For this review, take the finished solid that the model builds, in its own axes (mm). Give positions to 0.01 mm unless a question says otherwise; leave off trailing zeros. Order: outer loops, then holes, each group sorted by start corner. A loop starts at its lowest first (then second) coordinate and runs counter-clockwise, first axis right, second up. Notation, with made-up numbers: (37, 66) -> (44, 66) arc R18 cw to (44, 77) -> close; hole circle Ø3 at (67.5, 24). An arc over 180 degrees is marked (long way). Return JSON: item names as keys, results as strings. Group by question number.
1) Add section A-A (x = 4). Give the boundary of the cut face in (y, z).
2) Add section D-D (z = 2.75). Give the boundary of the cut face in (x, y).
3) Insertion check: P1, Ø3, axis at x = 3, y = 37.5, coming from the -Z side; P2, Ø3.5, axis at x = 38.5, y = 4, coming from the +Z side. Each pin has a flat end and moves straight along its axis. Give the tip position at first contact, or say it passes through.
4) Add section B-B (y = 38.5). Give the boundary of the cut face in (x, z), then the cut area to 3 significant figures.
5) Add section C-C (x = 47). Give the boundary of the cut face in (y, z), then the cut area to 3 significant figures.
6) To check wall thickness, follow line 1 along X through (y, z) = (4, 6.7); line 2 along X through (y, z) = (4, 5.55); line 3 along X through (y, z) = (38.5, 6.1). State the ranges of each line that lie inside material, in increasing order.
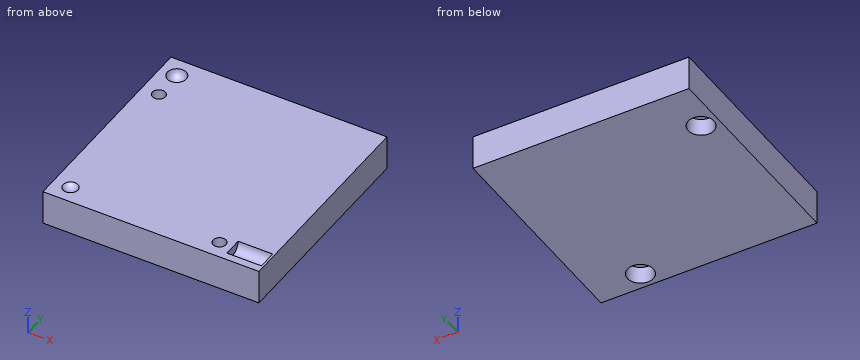
from build123d import *

# Parameters (mm, degrees)
CYLINDER012_R     = 2.2
CYLINDER012_DEPTH = 8
CYLINDER011_R     = 3
CYLINDER011_DEPTH = 4
CYLINDER010_R     = 1.5
CYLINDER010_DEPTH = 8
CYLINDER009_R     = 3
CYLINDER009_DEPTH = 4
CYLINDER008_R     = 1.5
CYLINDER008_DEPTH = 8
BOX002_W          = 50
BOX002_H          = 50
BOX002_DEPTH      = 8


with BuildPart() as cylinder012:
    # Cylinder012 → Cylinder012 (new body)
    with BuildSketch(Plane(origin=(41.5, 4, 8), x_dir=(0, 0, -1), z_dir=(1, 0, 0))):
        Circle(CYLINDER012_R)
    extrude(amount=CYLINDER012_DEPTH)


with BuildPart() as sphere003:
    # Sphere003 → Sphere003 (revolve)
    with BuildSketch(Plane(origin=(4, 45.5, 8.1), x_dir=(1, 0, 0), z_dir=(0, -1, 0))):
        with BuildLine():
            ThreePointArc((0, -2.2), (2.2, 0), (0, 2.2))
            Line((0, 2.2), (0, -2.2))
        make_face()
    revolve(axis=Axis((4, 45.5, 8.1), (0, 0, 1)))


with BuildPart() as sphere001:
    # Sphere001 → Sphere001 (revolve)
    with BuildSketch(Plane(origin=(4, 4, 9), x_dir=(1, 0, 0), z_dir=(0, -1, 0))):
        with BuildLine():
            ThreePointArc((0, -2), (2, 0), (0, 2))
            Line((0, 2), (0, -2))
        make_face()
    revolve(axis=Axis((4, 4, 9), (0, 0, 1)))


with BuildPart() as cylinder011:
    # Cylinder011 → Cylinder011 (new body)
    with BuildSketch(Plane.XY):
        Circle(CYLINDER011_R)
    extrude(amount=CYLINDER011_DEPTH)


with BuildPart() as springhole004:
    # Cylinder010 → Cylinder010 (new body)
    with BuildSketch(Plane.XY):
        Circle(CYLINDER010_R)
    extrude(amount=CYLINDER010_DEPTH)

    # Fusion005: union Cylinder011
    add(cylinder011.part)


with BuildPart() as springhole004_1:
    # Fusion005 placement: moved
    add(springhole004.part.moved(Location((4, 38.5, 0))))


with BuildPart() as cylinder009:
    # Cylinder009 → Cylinder009 (new body)
    with BuildSketch(Plane.XY):
        Circle(CYLINDER009_R)
    extrude(amount=CYLINDER009_DEPTH)


with BuildPart() as springhole003:
    # Cylinder008 → Cylinder008 (new body)
    with BuildSketch(Plane.XY):
        Circle(CYLINDER008_R)
    extrude(amount=CYLINDER008_DEPTH)

    # Fusion004: union Cylinder009
    add(cylinder009.part)


with BuildPart() as springhole003_1:
    # Fusion004 placement: moved
    add(springhole003.part.moved(Location((38.5, 4, 0))))


with BuildPart() as cut012:
    # Box002 → Box002 (new body)
    with BuildSketch(Plane.XY):
        with Locations((25, 25)):
            Rectangle(BOX002_W, BOX002_H)
    extrude(amount=BOX002_DEPTH)

    # Cut008: cut SpringHole003
    add(springhole003_1.part, mode=Mode.SUBTRACT)

    # Cut009: cut SpringHole004
    add(springhole004_1.part, mode=Mode.SUBTRACT)

    # Cut010: cut Sphere001
    add(sphere001.part, mode=Mode.SUBTRACT)

    # Cut011: cut Sphere003
    add(sphere003.part, mode=Mode.SUBTRACT)

    # Cut012: cut Cylinder012
    add(cylinder012.part, mode=Mode.SUBTRACT)


solid = cut012.part
Evaluation:
{
 "1": {"outline": "(0, 0) -> (35.5, 0) -> (35.5, 4) -> (37, 4) -> (37, 8) -> (5.73, 8) arc R2 cw to (2.27, 8) -> (0, 8) -> close; (40, 4) -> (41.5, 4) -> (41.5, 0) -> (50, 0) -> (50, 8) -> (47.7, 8) arc R2.2 cw to (43.3, 8) -> (40, 8) -> close"},
 "2": {"outline": "(0, 0) -> (50, 0) -> (50, 50) -> (0, 50) -> close; hole circle Ø6 at (4, 38.5); hole circle Ø6 at (38.5, 4)"},
 "3": {"P1": "z = 4", "P2": "z = 8"},
 "4": {"outline": "(0, 0) -> (1, 0) -> (1, 4) -> (2.5, 4) -> (2.5, 8) -> (0, 8) -> close; (5.5, 4) -> (7, 4) -> (7, 0) -> (50, 0) -> (50, 8) -> (5.5, 8) -> close", "area": "364 mm^2"},
 "5": {"outline": "(0, 0) -> (50, 0) -> (50, 8) -> (6.2, 8) arc R2.2 cw to (1.8, 8) -> (0, 8) -> close", "area": "392 mm^2"},
 "6": {"line 1": "0 to 37, 40 to 41.5, 49.5 to 50", "line 2": "0 to 37, 40 to 50", "line 3": "0 to 2.5, 5.5 to 50"}
}
